Autodesk Inventor part; units mm, degrees
ref_plane "Work Plane1" through (6, 2, 4.5) normal (0, 0, -1) x (-1, 0, 0)
ref_plane "Work Plane2" through (6, 2, -10.5) normal (0, 0, -1) x (-1, 0, 0)
ref_plane "YZ Plane" through (0, 0, 0) normal (1, 0, 0) x (0, 1, 0)
sketch "Sketch1" plane through (0, 0, 0) normal (0, 1, 0) x (-1, 0, 0)
  line L0 (8, 13.5) -> (-8, 13.5)
  line L1 (-8, 13.5) -> (-8, -13.5)
  line L2 (-8, -13.5) -> (8, -13.5)
  line L3 (8, -13.5) -> (8, 13.5)
  line L4 (8, 13.5) -> (-8, -13.5) construction
  line L5 (-8, 13.5) -> (8, -13.5) construction
  point P0 (0, 0)
  dimension "d0" = 16
  dimension "d1" = 27
extrude "Extrusion1" add sketch "Sketch1" along normal blind 2
sketch "Sketch2" plane through (0, 2, 0) normal (0, 1, 0) x (1, 0, 0)
  line L0 (8, 13.5) -> (-8, 13.5)
  line L1 (-6, 13.5) -> (6, 13.5)
  line L2 (6, 13.5) -> (6, -11.5)
  line L3 (6, -11.5) -> (-6, -11.5)
  line L4 (-6, -11.5) -> (-6, 13.5)
  line L5 (8, -13.5) -> (8, 13.5)
  line L6 (-8, 13.5) -> (-8, -13.5)
  line L7 (-8, -13.5) -> (8, -13.5)
  point P0 (0, 0)
  dimension "d4" = 2
  dimension "d5" = 2
  dimension "d6" = 2
extrude "Extrusion2" add sketch "Sketch2" along normal blind 3 contours L5 L7 L6 L0 L4 L3 L2
sketch "Sketch4" plane through (0, 5, 0) normal (0, 1, 0) x (1, 0, 0)
  line L0 (6, -11.5) -> (-6, -11.5)
  line L1 (-8, -13.5) -> (8, -13.5)
  line L2 (-6, -11.5) -> (6, -11.5)
  line L3 (6, -11.5) -> (6, -13.5)
  line L4 (6, -13.5) -> (-6, -13.5)
  line L5 (-6, -13.5) -> (-6, -11.5)
  line L6 (6, 13.5) -> (6, -11.5)
  point P0 (0, 0)
extrude "Extrusion3" add sketch "Sketch4" along normal blind 2
sketch "Sketch3" plane through (-8, 0, 13.5) normal (0, 0, 1) x (1, 0, 0)
  line L0 (14, 2) -> (2, 2) construction
  line L1 (2, 2) -> (14, 2) construction
  circle A0 centre (8, 7) radius 2.5
  line L2 (8, 11.4) -> (8, -1.9) construction
  line L3 (3.5, 7) -> (12.5, 7) construction
  circle A1 centre (3.5, 7) radius 1
  circle A2 centre (12.5, 7) radius 1
  line L4 (3.5, 8) -> (5.7087, 8)
  line L5 (12.5, 8) -> (10.2913, 8)
  line L6 (12.5, 6) -> (10.2913, 6)
  line L7 (5.7087, 6) -> (3.5, 6)
  point P0 (8, 0)
  dimension "d9" = 5
  dimension "d10" = 5
  dimension "d11" = 9
  dimension "d12" = 2
  dimension "d13" = 2
extrude "Extrusion4" cut sketch "Sketch3" against normal up to next
ref_plane "Work Plane1" through (6, 2, 4.5) normal (0, 0, -1) x (-1, 0, 0)
ref_plane "Work Plane2" through (6, 2, -10.5) normal (0, 0, -1) x (-1, 0, 0)
sketch "Sketch6" plane through (6, 2, 4.5) normal (0, 0, -1) x (-1, 0, 0)
  line L0 (-2, -2) -> (-2, 0)
  line L1 (-2, -2) -> (-2, 3)
  line L2 (-2, 0) -> (0, -2)
  line L3 (-2, -2) -> (14, -2)
  line L4 (0, -2) -> (-2, -2)
  line L5 (6, -3.4) -> (6, 6.4) construction
  line L6 (14, -2) -> (14, 0)
  line L7 (14, 0) -> (12, -2)
  line L8 (12, -2) -> (14, -2)
  point P0 (6, -2)
  dimension "d22" = 2
  dimension "d23" = 45
extrude "Extrusion5" cut sketch "Sketch6" along normal mid plane 3.6
sketch "Sketch7" plane through (6, 2, -10.5) normal (0, 0, -1) x (-1, 0, 0)
  line L0 (-2, 0) -> (0, -2)
  line L1 (-2, -2) -> (-2, 0)
  line L2 (0, -2) -> (-2, -2)
  line L3 (12, -2) -> (14, 0)
  line L4 (14, -2) -> (12, -2)
  line L5 (14, 0) -> (14, -2)
  point P0 (6, -2)
extrude "Extrusion6" cut sketch "Sketch7" against normal blind 3.6
sketch "Sketch8" plane through (0, 2, 0) normal (0, 1, 0) x (1, 0, 0)
  line L0 (-6, 13.5) -> (-6, -11.5)
  line L1 (6, -11.5) -> (6, 13.5)
  line L2 (-6, 13.5) -> (6, 13.5)
  line L3 (6, 13.5) -> (6, 11)
  line L4 (6, 11) -> (-6, 11)
  line L5 (-6, 11) -> (-6, 13.5)
  line L6 (-2.2913, -11.5) -> (2.2913, -11.5)
  point P0 (0, 0)
  point P1 (6, 13.5)
  point P2 (-6, 11)
  dimension "d28" = 22.5
extrude "Extrusion7" cut sketch "Sketch8" against normal up to next
sketch "Sketch9" plane through (0, 2, 0) normal (0, 1, 0) x (1, 0, 0)
  line L0 (-6, 11) -> (-6, -11.5)
  line L1 (6, -11.5) -> (6, 11)
  line L2 (-6, -10.5) -> (6, -10.5)
  line L3 (6, -10.5) -> (6, -7.3)
  line L4 (6, -7.3) -> (-6, -7.3)
  line L5 (-6, -7.3) -> (-6, -10.5)
  line L6 (-2.2913, -11.5) -> (2.2913, -11.5)
  point P0 (0, 0)
  point P1 (6, -10.5)
  dimension "d31" = 1
  dimension "d32" = 3.2
extrude "Extrusion8" cut sketch "Sketch9" against normal blind 1
equation "\"d5\" = d4"
equation "\"d6\" = d4"
properties part number "motor_top"
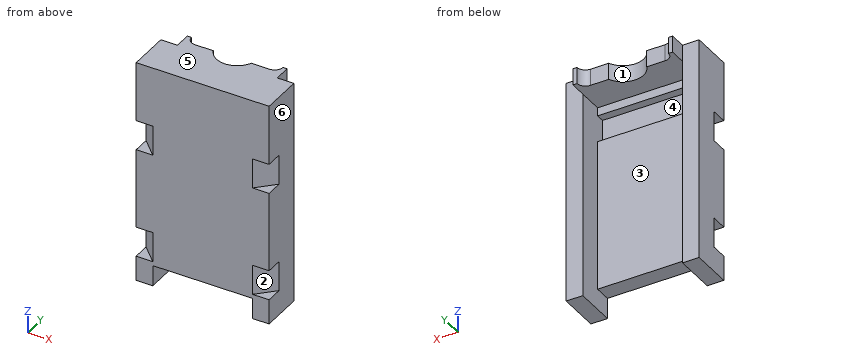
Could you check a few things on this model? Use its own coordinates, in mm. Face numbers are marked on the shaded views. A direction names the side the tool comes from. Give positions to 0.01 mm unless a question says otherwise; leave off trailing zeros. Loops run counter-clockwise (first coordinate to the right, second up) from the corner with the lowest first, then second, coordinate; pieces in that order, holes last. Notation, with made-up numbers: (-1.5, 21) -> (46.5, 21) arc R27 cw to (46.5, 55) -> close; hole circle Ø7 at (69.5, -3). An arc over 180 degrees is marked (long way). Answer as CSV lines item,"result". Start each with the question number.
(1) I need wall thicknesses on probe 1 along X at (y, z) = (3, 1.5); probe 2 along Y at (x, z) = (-1.75, -6.75); probe 3 along Y at (x, z) = (-7, 4). Which ranges of each line are inside material? Lowest first, please.
(2) If we section it at A-A on x = -2: Write out the boundary of the cut face in (y, z).
(3) Which directions (+Z, -Z, +X, -X, +Y, -Y) give clear straight access to the entire face, cutting with the end or side of a thin tool? Please do the marked faces 1, 2 and 3.
(4) If we section it at C-C on y = 3: Write out the boundary of the cut face in (x, z), then the cut area to 3 significant figures.
(5) If we section it at B-B on z = 0: Write out the boundary of the cut face in (x, y), then the cut area to 3 significant figures.
(6) If we section it at D-D on z = -9.75: Write out the boundary of the cut face in (x, y), then the cut area to 3 significant figures.
(7) I'm going to push flat-ended pins straight in: pin 1 Ø2.5 at (x, z) = (0, 9) entering from +Y; pin 2 Ø2 at (x, z) = (4, 12.5) entering from +Y; pin 3 Ø2 at (x, z) = (-7, 1.5) entering from +Y. Where does each tip first touch, or does it pass through?
(8) We'd pull the mould along Z, two halves only. Please class the marked faces 4, 5 and 6: released by +Z, released by -Z, zero draft, split by the parting line, or undercut.
Computed:
1,probe 1,"x = -8 to -6, 6 to 8"
1,probe 2,"y = 0 to 2"
1,probe 3,"y = 1 to 5"
2,outline,"(0, -11) -> (2, -11) -> (2, 7.3) -> (1, 7.3) -> (1, 10.5) -> (2, 10.5) -> (2, 11.5) -> (5.5, 11.5) -> (5.5, 13.5) -> (0, 13.5) -> close"
3,face 1,"+Z, -Z, +Y"
3,face 2,"+X, -Y"
3,face 3,"-Z, +Y"
4,outline,"(-8, -13.5) -> (-6, -13.5) -> (-6, 11.5) -> (6, 11.5) -> (6, -13.5) -> (8, -13.5) -> (8, 13.5) -> (-8, 13.5) -> close"
4,area,"132 mm2"
5,outline,"(-8, 0) -> (8, 0) -> (8, 5) -> (6, 5) -> (6, 2) -> (-6, 2) -> (-6, 5) -> (-8, 5) -> close"
5,area,"44.0 mm2"
6,outline,"(-8, 2) -> (-6, 0) -> (6, 0) -> (8, 2) -> (8, 5) -> (6, 5) -> (6, 2) -> (-6, 2) -> (-6, 5) -> (-8, 5) -> close"
6,area,"40.0 mm2"
7,pin 1,"stops at y = 1"
7,pin 2,"stops at y = 6.13"
7,pin 3,"stops at y = 5"
8,face 4,"undercut"
8,face 5,"released by +Z"
8,face 6,"zero draft"
